CAD build for the part. Positions are in the model's coordinates, mm. Round coordinates to 2 decimals unless told otherwise and drop trailing zeros. Order: outer loops, then holes, each group sorted by start corner. A loop starts at its lowest first (then second) coordinate and runs counter-clockwise, first axis right, second up. Notation, with made-up numbers: M -30,50.25 L -16,50.25 A23 cw -16,73.25 Z; hole C -0.5,47.5 d6. An arc over 180 degrees is marked long. Put each result on its own line as item: value.
Autodesk Inventor part; units mm, degrees
ref_plane "YZ Plane" through (0, 0, 0) normal (1, 0, 0) x (0, 1, 0)
ref_plane "XZ Plane" through (0, 0, 0) normal (0, 1, 0) x (-1, 0, 0)
ref_plane "XY Plane" through (0, 0, 0) normal (0, 0, 1) x (1, 0, 0)
sketch "Sketch1" plane through (0, 0, 0) normal (0, 0, 1) x (1, 0, 0)
  line L0 (0, 0) -> (160, 0)
  line L1 (160, 0) -> (160, 160)
  line L2 (160, 160) -> (0, 160)
  line L3 (0, 160) -> (0, 0)
  dimension "d0" = 160
  dimension "d1" = 160
extrude "Extrusion1" add sketch "Sketch1" along normal blind 10
sketch "Sketch2" plane through (0, 0, 10) normal (0, 0, 1) x (1, 0, 0)
  line L0 (0, 0) -> (160, 0)
  line L1 (0, 0) -> (15, 0)
  line L2 (15, 0) -> (15, 15)
  line L3 (160, 160) -> (0, 160)
  line L4 (0, 160) -> (15, 160)
  line L5 (15, 160) -> (15, 145)
  line L6 (160, 0) -> (160, 160)
  line L7 (160, 160) -> (145, 160)
  line L8 (145, 160) -> (145, 143.5)
  line L9 (160, 0) -> (160, 15)
  line L10 (160, 15) -> (145, 15)
  circle A0 centre (15, 145) radius 7.5
  circle A1 centre (145, 143.5) radius 7.5
  circle A2 centre (145, 15) radius 7.5
  circle A3 centre (15, 15) radius 7.5
  dimension "d4" = 15
  dimension "d5" = 15
  dimension "d6" = 15
  dimension "d7" = 15
  dimension "d8" = 15
  dimension "d9" = 16.5
  dimension "d10" = 15
  dimension "d11" = 15
  dimension "d12" = 15
  dimension "d13" = 15
  dimension "d14" = 15
  dimension "d15" = 15
extrude "Extrusion2" cut sketch "Sketch2" against normal blind 10
sketch "Sketch3" plane through (0, 0, 10) normal (0, 0, 1) x (1, 0, 0)
  line L0 (0, 160) -> (0, 0)
  line L1 (0, 0) -> (80, 0)
  line L2 (0, 0) -> (160, 0)
  line L3 (80, 0) -> (0, 0)
  line L4 (0, 0) -> (80, 0)
  dimension "d18" = 80
  dimension "d19" = 80
  dimension "d20" = 80
sketch "Sketch4" plane through (0, 0, 10) normal (0, 0, 1) x (1, 0, 0)
  line L0 (0, 0) -> (0, 80)
  line L1 (0, 160) -> (0, 0)
  line L2 (0, 80) -> (80, 80)
  circle A0 centre (80, 80) radius 7.5
  dimension "d21" = 80
  dimension "d22" = 80
  dimension "d23" = 15
extrude "Extrusion3" cut sketch "Sketch4" against normal blind 10
properties part number "106"
Item 1: Band-saw the part on C-C on z = 2.5. Give the cut face in (x, y), and give its area (3 significant figures).
Answers below:
outline: M 0,0 L 160,0 L 160,160 L 0,160 Z; hole C 15,15 d15; hole C 15,145 d15; hole C 80,80 d15; hole C 145,15 d15; hole C 145,143.5 d15
area: 24,700 mm²
Item 2: Band-saw the part on A-A on x = 15. Give the cut face in (y, z), and give its area (3 significant figures).
Answers below:
outline: M 0,0 L 7.5,0 L 7.5,10 L 0,10 Z; M 22.5,0 L 137.5,0 L 137.5,10 L 22.5,10 Z; M 152.5,0 L 160,0 L 160,10 L 152.5,10 Z
area: 1,300 mm²
Item 3: Probe line 1 along Y through (x, z) = (15, 7.5); line 2 along Y through (x, z) = (145, 4.25); line 3 along X through (y, z) = (143.5, 6.75). List the from-to ranges inside material, lowest first. Write a range as [from, to].
Answers below:
line 1: [0, 7.5], [22.5, 137.5], [152.5, 160]
line 2: [0, 7.5], [22.5, 136], [151, 160]
line 3: [0, 7.65], [22.35, 137.5], [152.5, 160]
Item 4: Band-saw the part on D-D on y = 80. Give the cut face in (x, z), and give its area (3 significant figures).
Answers below:
outline: M 0,0 L 72.5,0 L 72.5,10 L 0,10 Z; M 87.5,0 L 160,0 L 160,10 L 87.5,10 Z
area: 1,450 mm²
Item 5: Mould opens along Y. For faces 1 (the flat face through (79, 0, 5)), 2 (the flat face through (79, 99, 0)), 3 (the cylindrical face through (9.5, 20.1, 5.1)), 4 (the cylindrical face through (152.154, 17.253, 5.07)) say: pulls with the +Y half, pulls with the -Y half, needs draft (parallel to the pull), parting line crosses it, or undercut.
Answers below:
face 1: pulls with the -Y half
face 2: needs draft
face 3: undercut
face 4: undercut
